```python
from build123d import *

# Parameters (mm, degrees)
SKETCH2_W           = 30
SKETCH2_H           = 10
BOSS_EXTRUDE1_DEPTH = 100
SKETCH3_R           = 4
CUT_EXTRUDE1_DEPTH  = 30
FILLET1_R           = 5


with BuildPart() as part:
    # Sketch2 → Boss-Extrude1 (new body)
    with BuildSketch(Plane.XY):
        with Locations((15, 5)):
            Rectangle(SKETCH2_W, SKETCH2_H)
    extrude(amount=BOSS_EXTRUDE1_DEPTH)

    # Sketch3 → Cut-Extrude1 (cut)
    with BuildSketch(Plane(origin=(0, 10, 0), x_dir=(1, 0, 0), z_dir=(0, 1, 0))):
        with Locations(Location((15, -6, 0), (0, 0, 270))):
            Circle(SKETCH3_R)
    extrude(amount=-CUT_EXTRUDE1_DEPTH, mode=Mode.SUBTRACT)

    # Fillet1
    fillet1_edges = [part.edges().sort_by_distance(p)[0] for p in [
        (30, 5, 0),
    ]]
    fillet(fillet1_edges, radius=FILLET1_R)


solid = part.part
```
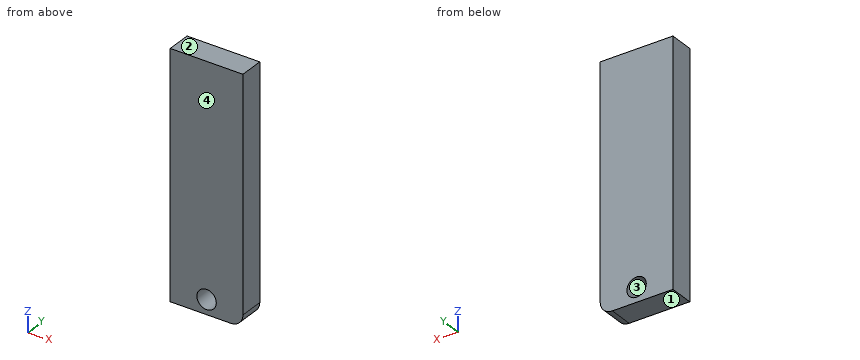
Could you check a few things on this model? Use its own coordinates, in mm. Face numbers are marked on the shaded views. Coordinates: 2 decimals unless noted, no trailing zeros. Loops run counter-clockwise (first coordinate to the right, second up) from the corner with the lowest first, then second, coordinate; pieces in that order, holes last.
1) Imagine slicing it at B-B (x = 15). List the corners of the cut face in (y, z) for me, and give its area (3 significant figures).
Reported:
outline: (0, 0) - (10, 0) - (10, 2) - (0, 2) - close; (0, 10) - (10, 10) - (10, 100) - (0, 100) - close
area: 920 mm2
2) Imagine slicing it at C-C (y = 3.75). List the corners of the cut face in (x, z) for me, and give its area (3 significant figures).
Reported:
outline: (0, 0) - (25, 0) arc R5 ccw to (30, 5) - (30, 100) - (0, 100) - close; hole circle Ø8 at (15, 6)
area: 2,940 mm2
3) Will this pin go through, and if not, where does the flat tip stop? pin 1 Ø3 at (x, z) = (22, 81.5) entering from -Y.
Reported:
pin 1: stops at y = 0
4) Thinking about a two-plate mould opening in Z: for the marked faces 1, 2, 3 and 4, which applies, released by +Z, released by -Z, zero draft, split by the parting line, or undercut?
Reported:
face 1: released by -Z
face 2: released by +Z
face 3: undercut
face 4: zero draft
5) Please list where these lines run through material, in increasing order: line 1 along X through (y, z) = (3, 6); line 2 along X through (y, z) = (1.5, 5); line 3 along Z through (x, y) = (26.25, 9.5).
Reported:
line 1: x = 0 to 11, 19 to 30
line 2: x = 0 to 11.13, 18.87 to 30
line 3: z = 0.16 to 100
6) Imagine slicing it at A-A (z = 6). List the corners of the cut face in (x, y) for me, and give its area (3 significant figures).
Reported:
outline: (0, 0) - (11, 0) - (11, 10) - (0, 10) - close; (19, 0) - (30, 0) - (30, 10) - (19, 10) - close
area: 220 mm2
